The model under review builds one solid part; all positions refer to its coordinate system, in mm. A direction names the side the tool comes from. Round coordinates to 2 decimals unless told otherwise and drop trailing zeros. Loops run counter-clockwise (first coordinate to the right, second up) from the corner with the lowest first, then second, coordinate; pieces in that order, holes last. Notation, with made-up numbers: (73, 78) - (116, 78) arc R26 ccw to (116, 94) - close; hole circle Ø8 at (68, 38). An arc over 180 degrees is marked (long way). Answer as CSV lines item,"result".
from build123d import *

# Parameters (mm, degrees)
CROQUIS1_R              = 25
CROQUIS1_R_2            = 11
SALIENTE_EXTRUIR1_DEPTH = 19
CROQUIS3_R              = 11
CROQUIS3_R_2            = 9.5
SALIENTE_EXTRUIR2_DEPTH = 13
SALIENTE_EXTRUIR3_START = -2
CROQUIS4_R              = 11
CROQUIS4_R_2            = 4
SALIENTE_EXTRUIR3_DEPTH = 2
SALIENTE_EXTRUIR4_START = -2.5
CROQUIS5_R              = 30
CROQUIS5_R_2            = 25
SALIENTE_EXTRUIR4_DEPTH = 2.5
CORTAR_EXTRUIR1_START   = 4
CROQUIS6_R              = 25
CROQUIS6_R_2            = 19
CORTAR_EXTRUIR1_DEPTH   = 4
SALIENTE_EXTRUIR5_REACH = 48.487
CROQUIS7_R              = 11
CROQUIS7_R_2            = 4
SALIENTE_EXTRUIR6_START = 1.5
CROQUIS8_R              = 6.1
CROQUIS8_R_2            = 4
SALIENTE_EXTRUIR6_DEPTH = 1.5
CROQUIS9_R              = 25
CROQUIS9_R_2            = 15
CORTAR_EXTRUIR2_DEPTH   = 1.5


with BuildPart() as part:
    # Croquis1 → Saliente-Extruir1 (new body)
    with BuildSketch(Plane.XY):
        Circle(CROQUIS1_R)
        Circle(CROQUIS1_R_2, mode=Mode.SUBTRACT)
    extrude(amount=SALIENTE_EXTRUIR1_DEPTH)

    # Croquis3 → Saliente-Extruir2 (add, through all)
    with BuildSketch(Plane(origin=(0, 0, 6), x_dir=(-1, 0, 0), z_dir=(0, 0, -1))):
        Circle(CROQUIS3_R)
        Circle(CROQUIS3_R_2, mode=Mode.SUBTRACT)
    extrude(amount=-SALIENTE_EXTRUIR2_DEPTH)

    # Croquis4 → Saliente-Extruir3 (add)
    with BuildSketch(Plane.XY.offset(19).offset(SALIENTE_EXTRUIR3_START)):
        with Locations(Location((0, 0, 0), (0, 0, 180))):
            Circle(CROQUIS4_R)
        Circle(CROQUIS4_R_2, mode=Mode.SUBTRACT)
    extrude(amount=SALIENTE_EXTRUIR3_DEPTH)

    # Croquis5 → Saliente-Extruir4 (add)
    with BuildSketch(Plane.XY.offset(19).offset(SALIENTE_EXTRUIR4_START)):
        Circle(CROQUIS5_R)
        Circle(CROQUIS5_R_2, mode=Mode.SUBTRACT)
    extrude(amount=SALIENTE_EXTRUIR4_DEPTH)

    # Croquis6 → Cortar-Extruir1 (cut)
    with BuildSketch(Plane(origin=(0, 0, 14.25), x_dir=(-1, 0, 0), z_dir=(0, 0, -1)).offset(CORTAR_EXTRUIR1_START)):
        Circle(CROQUIS6_R)
        Circle(CROQUIS6_R_2, mode=Mode.SUBTRACT)
    extrude(amount=-CORTAR_EXTRUIR1_DEPTH, mode=Mode.SUBTRACT)

    # Croquis7 → Saliente-Extruir5 (add, up to next)
    with BuildSketch(Plane(origin=(0, 0, 0), x_dir=(-1, 0, 0), z_dir=(0, 0, -1)), mode=Mode.PRIVATE) as saliente_extruir5_sk1:
        Circle(CROQUIS7_R)
        with Locations(Location((0, 0, 0), (0, 0, 180))):
            Circle(CROQUIS7_R_2, mode=Mode.SUBTRACT)
    saliente_extruir5_tool1 = extrude(saliente_extruir5_sk1.sketch, amount=-SALIENTE_EXTRUIR5_REACH, mode=Mode.PRIVATE) - part.part
    add(saliente_extruir5_tool1.solids().sort_by_distance((10.688873, 0, 0))[0])

    # Croquis8 → Saliente-Extruir6 (add)
    with BuildSketch(Plane(origin=(0, 0, 0), x_dir=(-1, 0, 0), z_dir=(0, 0, -1)).offset(SALIENTE_EXTRUIR6_START)):
        with Locations(Location((0, 0, 0), (0, 0, 180))):
            Circle(CROQUIS8_R)
        with Locations(Location((0, 0, 0), (0, 0, 180))):
            Circle(CROQUIS8_R_2, mode=Mode.SUBTRACT)
    extrude(amount=-SALIENTE_EXTRUIR6_DEPTH)

    # Croquis9 → Cortar-Extruir2 (cut)
    with BuildSketch(Plane(origin=(0, 0, 0), x_dir=(-1, 0, 0), z_dir=(0, 0, -1))):
        Circle(CROQUIS9_R)
        Circle(CROQUIS9_R_2, mode=Mode.SUBTRACT)
    extrude(amount=-CORTAR_EXTRUIR2_DEPTH, mode=Mode.SUBTRACT)


solid = part.part
1. Take a section at A-A (x = 0). State the section outline as (y, z) points.
Numbers:
outline,"(-30, 16.5) - (-25, 16.5) - (-25, 14.25) - (-19, 14.25) - (-19, 10.25) - (-25, 10.25) - (-25, 1.5) - (-15, 1.5) - (-15, 0) - (-6.1, 0) - (-6.1, -1.5) - (-4, -1.5) - (-4, 19) - (-30, 19) - close; (4, -1.5) - (6.1, -1.5) - (6.1, 0) - (15, 0) - (15, 1.5) - (25, 1.5) - (25, 10.25) - (19, 10.25) - (19, 14.25) - (25, 14.25) - (25, 16.5) - (30, 16.5) - (30, 19) - (4, 19) - close"
2. Wall thickness on probe 1 along Z at (x, y) = (20, 8.5); probe 2 along Y at (x, z) = (0, 17.75); probe 3 along Y at (x, z) = (0, 9.75): over which ranges is each line inside the solid? List them lowest first.
Numbers:
probe 1,"z = 1.5 to 10.25, 14.25 to 19"
probe 2,"y = -30 to -4, 4 to 30"
probe 3,"y = -25 to -4, 4 to 25"
3. Take a section at C-C (y = -7). State the section outline as (x, z) points, plus the area to 3 significant figures.
Numbers:
outline,"(-29.17, 16.5) - (-24, 16.5) - (-24, 14.25) - (-17.66, 14.25) - (-17.66, 10.25) - (-24, 10.25) - (-24, 1.5) - (-13.27, 1.5) - (-13.27, 0) - (13.27, 0) - (13.27, 1.5) - (24, 1.5) - (24, 10.25) - (17.66, 10.25) - (17.66, 14.25) - (24, 14.25) - (24, 16.5) - (29.17, 16.5) - (29.17, 19) - (-29.17, 19) - close"
area,"855 mm²"
4. Draft analysis for pull direction Z (two halves, no side actions). For faces 4 (the face through (-8.767, -16.856, 12.222)), 5 (the face through (4, 19, 10.25)), 6 (the face through (23.846, 7.509, 5.814)), 7 (the face through (1.3, 4, -1.5)), state which applies: +Z half, -Z half, draft (parallel to the pull), parting line (faces both ways), or undercut.
Numbers:
face 4,"undercut"
face 5,"undercut"
face 6,"draft"
face 7,"-Z half"
5. Clearance check with flat-ended pins moving along their axes: pin 1 (6 mm diameter, centred on x = -20, z = 2, fed in from -Y); pin 2 (1 mm diameter, centred on x = -14, z = 7, fed in from +Y); pin 3 (5 mm diameter, centred on x = -4, z = 5.5, fed in from +Y); pin 4 (7 mm diameter, centred on x = 0, y = 0, fed in from -Z). State where each tip first meets the part, or that it passes through.
Numbers:
pin 1,"stops at y = -18.33"
pin 2,"stops at y = 21.04"
pin 3,"stops at y = 24.95"
pin 4,"passes through"
6. Tool access review of faces 1 (the face through (-29.97, 1.32, 17.73)), 2 (the face through (4, 19, 14.25)), 3 (the face through (-6.094, -0.268, -0.76)): name each direction out of +Z, -Z, +X, -X, +Y, -Y from which nothing blocks a thin tool from reaching the whole face with its end or side.
Numbers:
face 1,"+Z, -Z"
face 2,"none"
face 3,"-Z"
7. Take a section at D-D (x = -17.5). State the section outline as (y, z) points.
Numbers:
outline,"(-24.37, 16.5) - (-17.85, 16.5) - (-17.85, 14.25) - (-7.4, 14.25) - (-7.4, 10.25) - (-17.85, 10.25) - (-17.85, 1.5) - (17.85, 1.5) - (17.85, 10.25) - (7.4, 10.25) - (7.4, 14.25) - (17.85, 14.25) - (17.85, 16.5) - (24.37, 16.5) - (24.37, 19) - (-24.37, 19) - close"
8. Take a section at B-B (y = -24). State the section outline as (x, z) points.
Numbers:
outline,"(-18, 16.5) - (-7, 16.5) - (-7, 14.25) - (7, 14.25) - (7, 16.5) - (18, 16.5) - (18, 19) - (-18, 19) - close; (-7, 1.5) - (7, 1.5) - (7, 10.25) - (-7, 10.25) - close"
